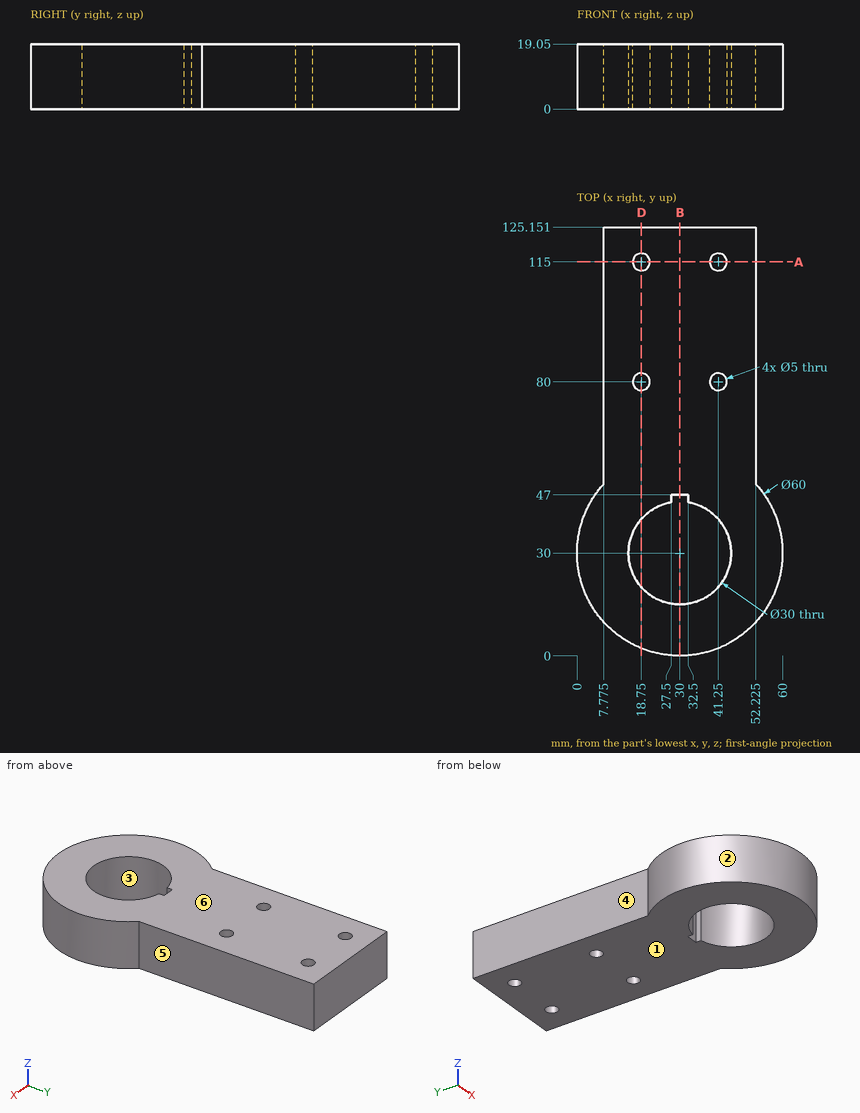
Source: three-view drawing plus pictorial views. Frame: mm from the lowest corner of the part. A direction names the side the tool comes from. Coordinates: 2 decimals unless noted, no trailing zeros. Order: outer loops, then holes, each group sorted by start corner. A loop starts at its lowest first (then second) coordinate and runs counter-clockwise, first axis right, second up. Notation, with made-up numbers: M 10.5,59 L 27.5,59 A35 ccw 27.5,97 Z; hole C -13,64.25 d6. An arc over 180 degrees is marked long. One line per question, with ' | ' between items. Start each with the question number.
Item 1: Pin query (flat end, axial travel): pin 1 Ø2 at (y, z) = (43, 7.5) entering from +X (1 decimal); pin 2 Ø3 at (y, z) = (18.5, 15.5) entering from -X; pin 3 Ø18 at (x, y) = (30, 30) entering from +Z; pin 4 Ø3 at (y, z) = (58, 11) entering from +X (3 decimals). Return the tip coordinate at first contact, or that it passes through.
Item 2: Ray query, probe 1 along Y at (x, z) = (41.25, 10); probe 2 along Y at (x, z) = (30, 12.5); probe 3 along Y at (x, z) = (41.5, 16.75). Return the intervals inside material, ascending. Write a range as [from, to].
Item 3: Draft query along X for the marked faces 1, 2, 3 and 4. Return one class per face: released by +X, released by -X, zero draft, split by the parting line, or undercut.
Item 4: Set-up query: the marked faces 5 and 6. Return all of +Z, -Z, +X, -X, +Y, -Y with unobstructed straight access to the full face (end or side cutting, diameter ignored); none if empty.
Item 5: Cut plane A-A, the plane y = 115. Count the separate pieces of the cut face and the enclosed holes in it, then the cut area to 3 significant figures.
Item 6: Cut plane B-B, the plane x = 30. Return the cut outline in (y, z).
Item 7: Cut plane D-D, the plane x = 18.75. Return the cut outline in (y, z), then the cut area to 3 significant figures.
A:
1) pin 1: stops at x = 57.5 | pin 2: stops at x = 1.72 | pin 3: passes through | pin 4: stops at x = 52.225
2) probe 1: y = [2.19, 20.08], [39.92, 77.5], [82.5, 112.5], [117.5, 125.15] | probe 2: y = [0, 15], [47, 125.15] | probe 3: y = [2.29, 20.37], [39.63, 77.51], [82.49, 112.51], [117.49, 125.15]
3) face 1: zero draft | face 2: split by the parting line | face 3: undercut | face 4: released by -X
4) face 5: +Z, -Z, +X, +Y | face 6: +Z, +X, -X, +Y, -Y
5) separate pieces: 3 | enclosed holes: 0 | area: 656 mm2
6) outline: M 0,0 L 15,0 L 15,19.05 L 0,19.05 Z; M 47,0 L 125.15,0 L 125.15,19.05 L 47,19.05 Z
7) outline: M 2.19,0 L 20.08,0 L 20.08,19.05 L 2.19,19.05 Z; M 39.92,0 L 77.5,0 L 77.5,19.05 L 39.92,19.05 Z; M 82.5,0 L 112.5,0 L 112.5,19.05 L 82.5,19.05 Z; M 117.5,0 L 125.15,0 L 125.15,19.05 L 117.5,19.05 Z | area: 1,770 mm2
